from build123d import *

# Parameters (mm, degrees)
BOSS_EXTRUDE1_DEPTH = 3.175


with BuildPart() as part:
    # Sketch1 → Boss-Extrude1 (new, symmetric)
    with BuildSketch(Plane(origin=(0, 0, 0), x_dir=(1, 0, 0), z_dir=(0, 1, 0))):
        with BuildLine():
            Line((-22.225, 82.944829198), (-22.225, -36.659057496))
            Line((-22.225, -36.659057496), (-49.38024545, -81.450315281))
            ThreePointArc((-49.38024545, -81.450315281), (0, -95.25), (49.38024545, -81.450315281))
            Line((49.38024545, -81.450315281), (22.225, -36.659057496))
            Line((22.225, -36.659057496), (22.225, 82.944829198))
            Line((22.225, 82.944829198), (29.583016855, 110.405321945))
            ThreePointArc((29.583016855, 110.405321945), (0, 114.3), (-29.583016855, 110.405321945))
            Line((-29.583016855, 110.405321945), (-22.225, 82.944829198))
        make_face()
    extrude(amount=BOSS_EXTRUDE1_DEPTH, both=True)


solid = part.part
Work out the finished part from the listing and answer in its coordinate system (mm). A direction names the side the tool comes from. Give positions to 0.01 mm unless a question says otherwise; leave off trailing zeros. Write each loop counter-clockwise with the first axis right and the second up, starting at its lowest first coordinate (ties: lowest second). Pieces come first, ordered by that corner, then holes. Notation, with made-up numbers: (-23, 31) - (17, 31) arc R15 ccw to (17, 59) - close; hole circle Ø4 at (-11, -12). An arc over 180 degrees is marked (long way). One line per item, written item: value. Start each with the question number.
1. Consider probe 1 along X at (y, z) = (0.5, -77) (3 decimals); probe 2 along Z at (x, y) = (-2, -0.75); probe 3 along X at (y, z) = (2.5, 82). Determine where each line is inside the solid, lowest interval first.
2. Given pin 1 (3 mm diameter, centred on y = -1.5, z = 31.5, fed in from -X) (3 decimals), flat-ended and moving along its own axis, determine where the tip first touches the part or whether it passes through.
3. For faces 5 (the flat face through (-1, -3.175, 12)), 6 (the flat face through (-22.225, 0, -24)), 7 (the flat face through (25.85, 0.04, -96.48)), determine the directions among +Z, -Z, +X, -X, +Y, -Y from which every point of the face is accessible in a straight line to the end or side of a thin tool.
4. Find section A-A (y = -0.5). Write down the section's boundary in (x, z) (3 decimals), then the cut area to 3 significant figures.
5. For a pull along Z with two mould halves and no side action, classify faces 1 (the flat face through (35.993, 0.044, 59.368)), 2 (the flat face through (-1, 3.175, 12)), 3 (the flat face through (-35.61, 0.04, 58.74)), 4 (the cylindrical face through (0.4, 0, -114.3)) as +Z half, -Z half, draft (parallel to the pull), parting line (faces both ways), or undercut.
6. Find section B-B (z = 30.5). Write down the section's boundary in (x, y) (3 decimals).
7. Find section C-C (x = 33.5). Write down the section's boundary in (y, z) (3 decimals).
Geometry results:
1. probe 1: -22.225 to 22.225
1. probe 2: -114.28 to 95.23
1. probe 3: -48.46 to 48.46
2. pin 1: x = -22.225
3. face 5: +Z, -Z, +X, -X, -Y
3. face 6: -X, +Y, -Y
3. face 7: +X, +Y, -Y
4. outline: (-49.38, 81.45) - (-22.225, 36.659) - (-22.225, -82.945) - (-29.583, -110.405) arc R114.3 ccw to (29.583, -110.405) - (22.225, -82.945) - (22.225, 36.659) - (49.38, 81.45) arc R95.25 ccw to start
4. area: 11,000 mm2
5. face 1: undercut
5. face 2: draft
5. face 3: undercut
5. face 4: -Z half
6. outline: (-22.225, -3.175) - (22.225, -3.175) - (22.225, 3.175) - (-22.225, 3.175) - close
7. outline: (-3.175, 55.257) - (3.175, 55.257) - (3.175, 89.165) - (-3.175, 89.165) - close
